Check sheet for the modelled part. Datum: model origin and axes. Units: mm. Face numbers are marked on the shaded views. Round coordinates to 2 decimals unless told otherwise and drop trailing zeros. Write each loop counter-clockwise with the first axis right and the second up, starting at its lowest first coordinate (ties: lowest second). Pieces come first, ordered by that corner, then holes. Notation, with made-up numbers: (81, -37) - (102, -37) arc R23 cw to (102, -15) - close; hole circle Ø11 at (-12, 28). An arc over 180 degrees is marked (long way). Answer as a JSON object with one key per item and string values. Group by question number.
Item 1: Sectioned sample at A-A on x = 0. Record the boundary of the cut face in (y, z).
Item 2: Release check for a two-part mould opening along X. For the marked faces 1 and 2 record: pulls with the +X half, pulls with the -X half, needs draft (parallel to the pull), parting line crosses it, or undercut.
Item 3: Thickness scan on line 1 (Y direction, x = 0, z = 0.95); line 2 (X direction, y = -5.75, z = 2); line 3 (X direction, y = 2.75, z = 0.7). Record the ranges inside material, lowest first.
Item 4: Sectioned sample at C-C on x = -4.5. Record the boundary of the cut face in (y, z) (3 decimals), plus the area to 3 significant figures.
Item 5: Sectioned sample at B-B on y = 0. Record the boundary of the cut face in (x, z) (3 decimals).
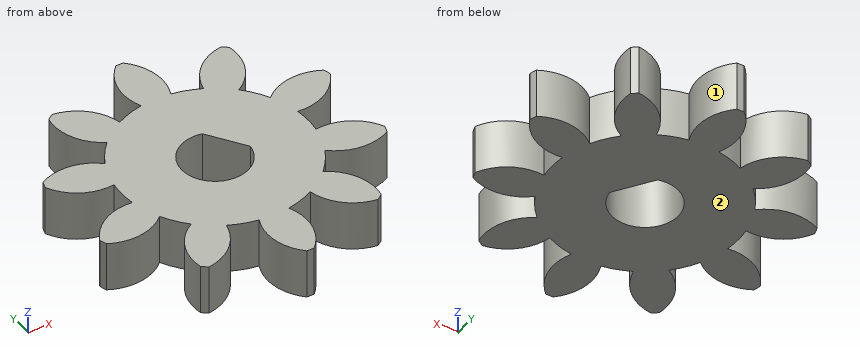
```python
from build123d import *

# Parameters (mm, degrees)
SKETCH1_R           = 9
BOSS_EXTRUDE1_DEPTH = 3
CUT_EXTRUDE1_DEPTH  = 14.076696831
CIRPATTERN1_COUNT   = 10
CUT_EXTRUDE4_DEPTH  = 13.821408374


with BuildPart() as part:
    # Sketch1 → Boss-Extrude1 (new body)
    with BuildSketch(Plane.XY):
        Circle(SKETCH1_R)
    extrude(amount=BOSS_EXTRUDE1_DEPTH)

    # Sketch2 → Cut-Extrude1 (cut, through all)
    with BuildSketch(Plane.XY.offset(3)):
        with BuildLine():
            ThreePointArc((5.110667533, 7.408176386), (3.438910397, 6.629232039), (2.538761327, 5.019493592))
            ThreePointArc((2.538761327, 5.019493592), (1.738220593, 5.349692904), (0.896483249, 5.553102087))
            ThreePointArc((0.896483249, 5.553102087), (1.114427873, 7.384502195), (0.21979994, 8.997315599))
            ThreePointArc((0.21979994, 8.997315599), (2.781152949, 8.559508647), (5.110667533, 7.408176386))
        make_face()
    cut_extrude1 = extrude(amount=-CUT_EXTRUDE1_DEPTH, mode=Mode.SUBTRACT)

    # CirPattern1: Cut-Extrude1 ×10 about axis
    cirpattern1_axis = Axis((0, 0, 0), (0, 0, 1))
    for i in range(1, CIRPATTERN1_COUNT):
        add(cut_extrude1.rotate(cirpattern1_axis, i * 360 / CIRPATTERN1_COUNT), mode=Mode.SUBTRACT)

    # Sketch5 → Cut-Extrude4 (cut, through all)
    with BuildSketch(Plane.XY.offset(3)):
        with BuildLine():
            Line((1.985580324, -0.239730633), (0.486047904, 1.940040575))
            ThreePointArc((0.486047904, 1.940040575), (-1.647752152, -1.133539961), (1.985580324, -0.239730633))
        make_face()
    extrude(amount=-CUT_EXTRUDE4_DEPTH, mode=Mode.SUBTRACT)


solid = part.part
```
Completed:
{
 "1": {"outline": "(-9, 0) - (-2, 0) - (-2, 3) - (-9, 3) - close; (2, 0) - (9, 0) - (9, 3) - (2, 3) - close"},
 "2": {"face 1": "undercut", "face 2": "needs draft"},
 "3": {"line 1": "-9 to -2, 2 to 9", "line 2": "-5.4 to -2.79, -0.98 to 0.98, 2.79 to 5.4", "line 3": "-8.57 to -5.22, -4.91 to 4.91, 5.22 to 8.57"},
 "4": {"outline": "(-7.266, 0) - (-4.327, 0) - (-4.327, 3) - (-7.266, 3) - close; (-3.375, 0) - (3.375, 0) - (3.375, 3) - (-3.375, 3) - close; (4.327, 0) - (7.266, 0) - (7.266, 3) - (4.327, 3) - close", "area": "37.9 mm²"},
 "5": {"outline": "(-5.625, 0) - (-2, 0) - (-2, 3) - (-5.625, 3) - close; (1.821, 0) - (5.625, 0) - (5.625, 3) - (1.821, 3) - close"}
}
